Could you check a few things on this drawing? It's one solid part, dimensions in mm from its lowest x, y, z. Give positions to 0.01 mm unless a question says otherwise; leave off trailing zeros. Order: outer loops, then holes, each group sorted by start corner. A loop starts at its lowest first (then second) coordinate and runs counter-clockwise, first axis right, second up.
Item 1: I'm going to push flat-ended pins straight in: pin 1 Ø2 at (x, y) = (31.04, 15.27) entering from +Z; pin 2 Ø1.6 at (x, z) = (23, 2) entering from +Y; pin 3 Ø1.6 at (x, z) = (9.5, 1.5) entering from -Y (3 decimals); pin 4 Ø1 at (y, z) = (53.5, 1.5) entering from -X. Where does each tip first touch, or does it pass through?
Item 2: I want a section at D-D, the plane x = 3.5. Write out the boundary of the cut face in (y, z) (1 decimal), then the cut area to 3 significant figures.
Item 3: If I drill on line 1 along X through (y, z) = (30.5, 2.95); line 2 along Y through (x, z) = (30.5, 0.45) (1 decimal); line 3 along X through (y, z) = (37, 2.4) (1 decimal), over which ranges is the centre line in solid material (lowest first)?
Item 4: I want a section at A-A, the plane y = 50. Write out the boundary of the cut face in (x, z) (1 decimal).
Item 5: I want a section at B-B, the plane x = 14. Write out the boundary of the cut face in (y, z) (1 decimal).
Item 6: I want a section at C-C, the plane z = 1.75. Write out the boundary of the cut face in (x, y) (1 decimal).
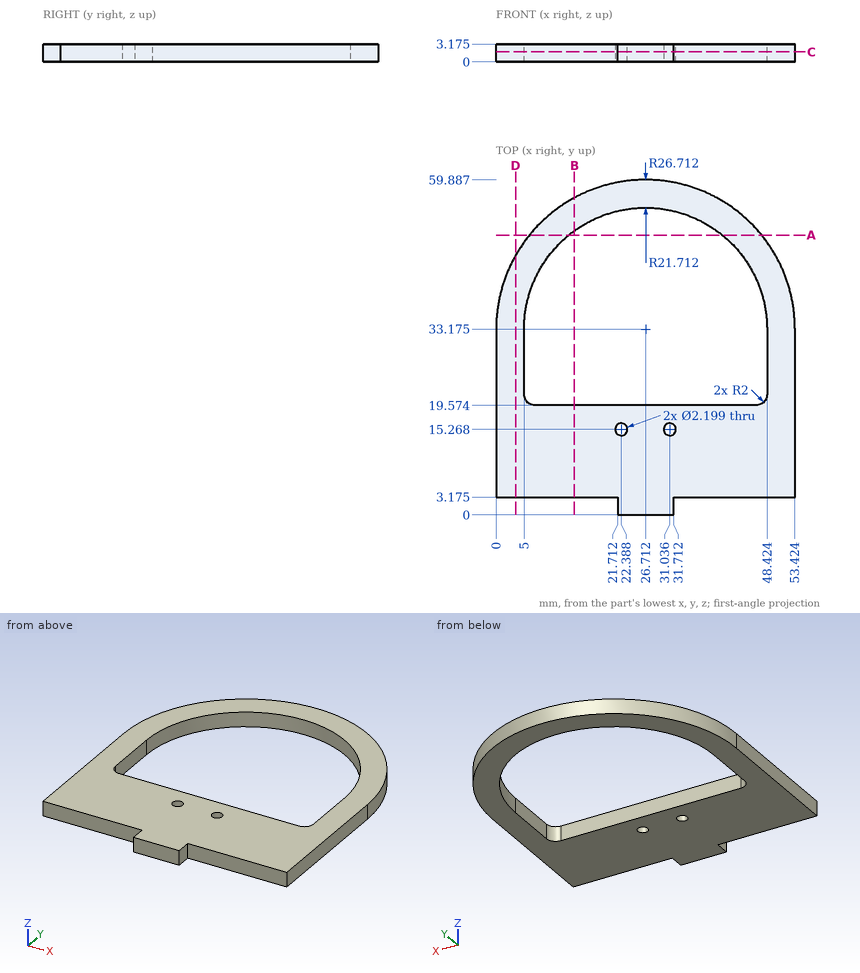
Results list:
1. pin 1: passes through
1. pin 2: stops at y = 59.73
1. pin 3: stops at y = 3.175
1. pin 4: stops at x = 8.81
2. outline: (3.2, 0) - (46.4, 0) - (46.4, 3.2) - (3.2, 3.2) - close
2. area: 137 mm2
3. line 1: x = 0 to 5, 48.42 to 53.42
3. line 2: y = 0 to 14.3, 16.2 to 19.6, 54.6 to 59.6
3. line 3: x = 0.3 to 5.3, 48.1 to 53.1
4. outline: (6, 0) - (13, 0) - (13, 3.2) - (6, 3.2) - close; (40.4, 0) - (47.5, 0) - (47.5, 3.2) - (40.4, 3.2) - close
5. outline: (3.2, 0) - (19.6, 0) - (19.6, 3.2) - (3.2, 3.2) - close; (50.8, 0) - (56.7, 0) - (56.7, 3.2) - (50.8, 3.2) - close
6. outline: (0, 3.2) - (21.7, 3.2) - (21.7, 0) - (31.7, 0) - (31.7, 3.2) - (53.4, 3.2) - (53.4, 33.2) arc R26.7 ccw to (0, 33.2) - close; hole (5, 21.6) arc R2 ccw to (7, 19.6) - (46.4, 19.6) arc R2 ccw to (48.4, 21.6) - (48.4, 33.2) arc R21.7 ccw to (5, 33.2) - close; hole circle Ø2.2 at (22.4, 15.3); hole circle Ø2.2 at (31, 15.3)
